Read the model definition and answer for the solid it produces. Units are mm, in the model's axes. Face numbers are marked on the shaded views. A direction names the side the tool comes from. Coordinates: 2 decimals unless noted, no trailing zeros. Write each loop counter-clockwise with the first axis right and the second up, starting at its lowest first coordinate (ties: lowest second). Pieces come first, ordered by that corner, then holes. Notation, with made-up numbers: (-17, -31.75) -> (5, -31.75) arc R18 ccw to (5, -12.75) -> close; hole circle Ø6 at (65, 9). An arc over 180 degrees is marked (long way). Write item = value, one per line. Start each with the question number.
1) Find the intervals of material crossed by line 1 along X through (y, z) = (-25, 21.5); line 2 along X through (y, z) = (16.5, 12); line 3 along Z through (x, y) = (-14, -26.5), in increasing order. Write a range as from..to.
2) Section C-C (x = -42.5) is taken. Determine the outline of the cut face in (y, z), plus the area to 3 significant figures.
3) A tool of negligible diameter and unlimited length cuts with its end or side. For the marked faces 4, 5 and 6, from which of +Z, -Z, +X, -X, +Y, -Y can it reach the whole face along a straight path? Write none if from no direction.
4) Section D-D (z = 7) is taken. Determine the outline of the cut face in (x, y).
5) Section A-A (z = 25) is taken. Determine the outline of the cut face in (x, y) (3 decimals).
6) Flat-ended cylindrical pins translate along their axes: pin 1 Ø8 at (x, y) = (-22.5, -9.5) entering from -Z; pin 2 Ø3 at (x, y) = (-8, -13.5) entering from +Z; pin 3 Ø7.5 at (x, y) = (-2.5, 16.5) entering from +Z. Find the tip coordinate at first contact, or state that the pin passes through.
7) Section B-B (y = -0.5) is taken. Determine the outline of the cut face in (x, z) (3 decimals).
8) For a pull along X with two mould halves and no side action, classify the marked faces 1, 2 and 3 as released by +X, released by -X, zero draft, split by the parting line, or undercut.
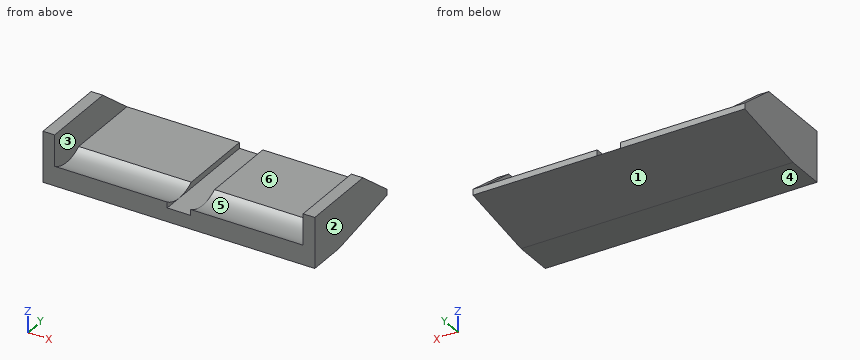
from build123d import *

# Parameters (mm, degrees)
F0_W      = 177.8
F0_H      = 76.2
F1_DEPTH  = 12.7
F3_DEPTH  = 197.612
F4_W      = 7.62
F4_H      = 76.2
F5_DEPTH  = 20.32
F6_W      = 7.62
F6_H      = 76.2
F7_DEPTH  = 20.32
F9_DEPTH  = 73.66
F11_DEPTH = 73.66
F13_DEPTH = 228.6
F15_DEPTH = 228.6


with BuildPart() as f1:
    # F0 (on Top) → F1 (new body)
    with BuildSketch(Plane.XY):
        Rectangle(F0_W, F0_H)
    extrude(amount=F1_DEPTH)

    # F2 (on face) → F3 (cut)
    with BuildSketch(Plane.XZ.offset(38.1)):
        Polygon((-7.62, 8.89), (0, 8.89), (7.62, 8.89), (7.62, 12.7), (-7.62, 12.7), align=None)
    extrude(amount=-F3_DEPTH, mode=Mode.SUBTRACT)

    # F4 (on face) → F5 (join)
    with BuildSketch(Plane.XY.offset(12.7)):
        with Locations((-85.09, 0)):
            Rectangle(F4_W, F4_H)
    extrude(amount=F5_DEPTH)

    # F6 (on face) → F7 (join)
    with BuildSketch(Plane.XY.offset(12.7)):
        with Locations((85.09, 0)):
            Rectangle(F6_W, F6_H)
    extrude(amount=F7_DEPTH)

    # F8 (on face) → F9 (cut)
    with BuildSketch(Plane.YZ.offset(-7.62)):
        with BuildLine():
            Line((-12.7, 12.7), (-38.1, 12.7))
            ThreePointArc((-38.1, 12.7), (-25.4, 8.898353), (-12.7, 12.7))
        make_face()
    extrude(amount=-F9_DEPTH, mode=Mode.SUBTRACT)

    # F10 (on face) → F11 (cut)
    with BuildSketch(Plane(origin=(7.62, 0, 0), x_dir=(0, -1, 0), z_dir=(-1, 0, 0))):
        with BuildLine():
            ThreePointArc((12.7, 12.7), (25.4, 8.898353), (38.1, 12.7))
            Line((38.1, 12.7), (12.7, 12.7))
        make_face()
    extrude(amount=-F11_DEPTH, mode=Mode.SUBTRACT)

    # F12 (on face) → F13 (cut)
    with BuildSketch(Plane(origin=(-88.9, 0, 0), x_dir=(0, -1, 0), z_dir=(-1, 0, 0))):
        Polygon((-38.1, 0), (12.7, 0), (-38.1, 8.89), align=None)
    extrude(amount=-F13_DEPTH, mode=Mode.SUBTRACT)

    # F14 (on face) → F15 (cut)
    with BuildSketch(Plane.YZ.offset(88.9)):
        Polygon((38.1, 33.02), (12.7, 33.02), (38.1, 12.7), align=None)
    extrude(amount=-F15_DEPTH, mode=Mode.SUBTRACT)


solid = f1.part
Answer key:
q1.line_1 = -88.9..-81.28, 81.28..88.9
q1.line_2 = -88.9..-7.62, 7.62..88.9
q1.line_3 = 0..8.92
q2.outline = (-38.1, 0) -> (-12.7, 0) -> (38.1, 8.89) -> (38.1, 12.7) -> (-12.7, 12.7) arc R23.11 cw to (-38.1, 12.7) -> close
q2.area = 676 mm^2
q3.face_4 = -Z, +X, -X, +Y, -Y
q3.face_5 = +Z
q3.face_6 = +Z, +Y, -Y
q4.outline = (-88.9, -38.1) -> (88.9, -38.1) -> (88.9, 27.3) -> (-88.9, 27.3) -> close
q5.outline = (-88.9, -38.1) -> (-81.28, -38.1) -> (-81.28, 22.725) -> (-88.9, 22.725) -> close; (81.28, -38.1) -> (88.9, -38.1) -> (88.9, 22.725) -> (81.28, 22.725) -> close
q6.pin_1 = 0
q6.pin_2 = 12.7
q6.pin_3 = 8.89
q7.outline = (-88.9, 2.135) -> (88.9, 2.135) -> (88.9, 33.02) -> (81.28, 33.02) -> (81.28, 12.7) -> (7.62, 12.7) -> (7.62, 8.89) -> (-7.62, 8.89) -> (-7.62, 12.7) -> (-81.28, 12.7) -> (-81.28, 33.02) -> (-88.9, 33.02) -> close
q8.face_1 = zero draft
q8.face_2 = released by +X
q8.face_3 = undercut
